```python
from build123d import *

# Parameters (mm, degrees)
SKETCH_1_W          = 40
SKETCH_1_H          = 40
SKETCH_1_W_2        = 38
SKETCH_1_H_2        = 38
EXTRUDE_1_DEPTH     = 295
SKETCH_3_R          = 1.6
CUT_EXTRUDE_2_DEPTH = 60


with BuildPart() as part:
    # 草图1 → 凸台-拉伸1 (new, symmetric)
    with BuildSketch(Plane.XY):
        Rectangle(SKETCH_1_W, SKETCH_1_H)
        Rectangle(SKETCH_1_W_2, SKETCH_1_H_2, mode=Mode.SUBTRACT)
    extrude(amount=EXTRUDE_1_DEPTH, both=True)

    # 草图3 → 切除-拉伸2 (cut)
    with BuildSketch(Plane(origin=(0, 20, 0), x_dir=(1, 0, 0), z_dir=(0, 1, 0))):
        with Locations(Location((-10, 245, 0), (0, 0, 270))):
            Circle(SKETCH_3_R)
        with Locations(Location((10, 245, 0), (0, 0, 270))):
            Circle(SKETCH_3_R)
        with Locations(Location((10, 265, 0), (0, 0, 270))):
            Circle(SKETCH_3_R)
        with Locations(Location((-10, 265, 0), (0, 0, 270))):
            Circle(SKETCH_3_R)
        with Locations(Location((-10, 285, 0), (0, 0, 270))):
            Circle(SKETCH_3_R)
        with Locations(Location((10, 285, 0), (0, 0, 270))):
            Circle(SKETCH_3_R)
        with Locations(Location((10, -285, 0), (0, 0, 270))):
            Circle(SKETCH_3_R)
        with Locations(Location((-10, -285, 0), (0, 0, 270))):
            Circle(SKETCH_3_R)
        with Locations(Location((-10, -265, 0), (0, 0, 270))):
            Circle(SKETCH_3_R)
        with Locations(Location((10, -265, 0), (0, 0, 270))):
            Circle(SKETCH_3_R)
        with Locations(Location((10, -245, 0), (0, 0, 270))):
            Circle(SKETCH_3_R)
        with Locations(Location((-10, -245, 0), (0, 0, 270))):
            Circle(SKETCH_3_R)
    extrude(amount=-CUT_EXTRUDE_2_DEPTH, mode=Mode.SUBTRACT)


solid = part.part
```
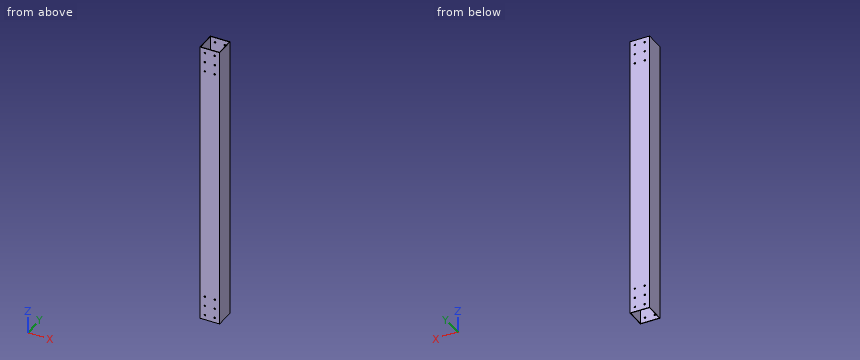
Input: part model. Units: mm. Frame: model coordinates. Give positions to 0.01 mm unless a question says otherwise; leave off trailing zeros. Order: outer loops, then holes, each group sorted by start corner. A loop starts at its lowest first (then second) coordinate and runs counter-clockwise, first axis right, second up. Notation, with made-up numbers: (34, 73.5) - (70, 73.5) arc R13 cw to (70, 82.5) - close; hole circle Ø4 at (64.5, 79). An arc over 180 degrees is marked (long way). One line per item, written item: value.
1. Cut plane C-C, the plane z = 91.5. Output: boundary loops of the cut face in (x, y), and give its area (3 significant figures).
Determined:
outline: (-20, -20) - (20, -20) - (20, 20) - (-20, 20) - close; hole (-19, -19) - (19, -19) - (19, 19) - (-19, 19) - close
area: 156 mm2
2. Pin query (flat end, axial travel): pin 1 Ø2.5 at (x, z) = (-10, -245) entering from -Y. Return the tip coordinate at first contact, or that it passes through.
Determined:
pin 1: through
3. Cut plane A-A, the plane y = -0.5. Output: boundary loops of the cut face in (x, z), and give its area (3 significant figures).
Determined:
outline: (-20, -295) - (-19, -295) - (-19, 295) - (-20, 295) - close; (19, -295) - (20, -295) - (20, 295) - (19, 295) - close
area: 1,180 mm2
4. Line query: probe 1 along X at (y, z) = (-19.7, -265); probe 2 along X at (y, z) = (1, 183.5). Output: solid intervals per line, ascending.
Determined:
probe 1: -20 to -11.6, -8.4 to 8.4, 11.6 to 20
probe 2: -20 to -19, 19 to 20
